For this review, take the finished solid that the model builds, in its own axes (mm). A direction names the side the tool comes from. Coordinates: 2 decimals unless noted, no trailing zeros. Loops run counter-clockwise (first coordinate to the right, second up) from the corner with the lowest first, then second, coordinate; pieces in that order, holes last.
1. Take a section at A-A, the plane x = -106. State the section outline as (y, z) points.
2. Take a section at B-B, the plane z = 183.5. State the section outline as (x, y) points.
3. To check wall thickness, follow probe 1 along Z at (x, y) = (-83, 1.75); probe 2 along X at (y, z) = (15, 168); probe 3 along Y at (x, z) = (-171, 224). State the ranges of each line that lie inside material, in increasing order.
4. Clearance check with a flat-ended pin moving along its axis: P1, Ø8, axis at x = -85, z = 205, coming from the -Y side. State where the tip first meets the part, or that it passes through.
5. Take a section at C-C, the plane y = 13.75. State the section outline as (x, z) points.
6. Mouldability with a two-part tool opening along X and no side actions: class faces 3 (the face through (-182, 13, 134)), 4 (the face through (-179, 12, 134)), 5 (the face through (-6, 12, 131)), 6 (the face through (-91, 13, 3)) as pulls with the +X half, pulls with the -X half, needs draft (parallel to the pull), parting line crosses it, or undercut.
7. Machinability: for faces 1 (the face through (-94, 12, 259)), 2 (the face through (-91, 13, 262)), which of the approach directions +Z, -Z, +X, -X, +Y, -Y give a long, thin tool a straight path to every point of the face, cutting with its end or side? Answer none if there is none.
Autodesk Inventor part; units mm, degrees
ref_plane "YZ Plane" through (0, 0, 0) normal (1, 0, 0) x (0, 1, 0)
ref_plane "XZ Plane" through (0, 0, 0) normal (0, 1, 0) x (-1, 0, 0)
ref_plane "XY Plane" through (0, 0, 0) normal (0, 0, 1) x (1, 0, 0)
sketch "Esboço1" plane through (0, 0, 0) normal (0, 1, 0) x (-1, 0, 0)
  line L0 (3, 3) -> (182, 3)
  line L1 (3, 262) -> (182, 262)
  line L2 (182, 262) -> (182, 3)
  line L3 (182, 3) -> (3, 3)
  line L4 (3, 3) -> (3, 262)
  line L5 (6, 6) -> (179, 6)
  line L6 (179, 259) -> (6, 259)
  line L7 (179, 6) -> (6, 6)
  line L8 (6, 6) -> (6, 259)
  line L9 (6, 259) -> (179, 259)
  line L10 (179, 259) -> (179, 6)
  point P0 (0, 0)
  point P1 (0, 0)
extrude "Extrusão1" add sketch "Esboço1" along normal blind 25
sketch "Esboço2" plane through (0, 25, 0) normal (0, 1, 0) x (1, 0, 0)
  line L0 (-182, -3) -> (-3, -3)
  line L1 (-3, -262) -> (-3, -3)
  line L2 (-182, -3) -> (-3, -3)
  line L3 (-3, -3) -> (-3, -262)
  line L4 (-3, -262) -> (-182, -262)
  line L5 (-182, -262) -> (-182, -3)
  point P0 (0, 0)
extrude "Extrusão2" add sketch "Esboço2" along normal blind 2
properties part number "tampa caixa" material "PCL plástico"
Results list:
1. outline: (0, 3) - (27, 3) - (27, 262) - (0, 262) - (0, 259) - (25, 259) - (25, 6) - (0, 6) - close
2. outline: (-182, 0) - (-179, 0) - (-179, 25) - (-6, 25) - (-6, 0) - (-3, 0) - (-3, 27) - (-182, 27) - close
3. probe 1: z = 3 to 6, 259 to 262
3. probe 2: x = -182 to -179, -6 to -3
3. probe 3: y = 25 to 27
4. P1: stops at y = 25
5. outline: (-182, 3) - (-3, 3) - (-3, 262) - (-182, 262) - close; hole (-179, 6) - (-6, 6) - (-6, 259) - (-179, 259) - close
6. face 3: pulls with the -X half
6. face 4: undercut
6. face 5: undercut
6. face 6: needs draft
7. face 1: -Y
7. face 2: +Z, +X, -X, +Y, -Y
